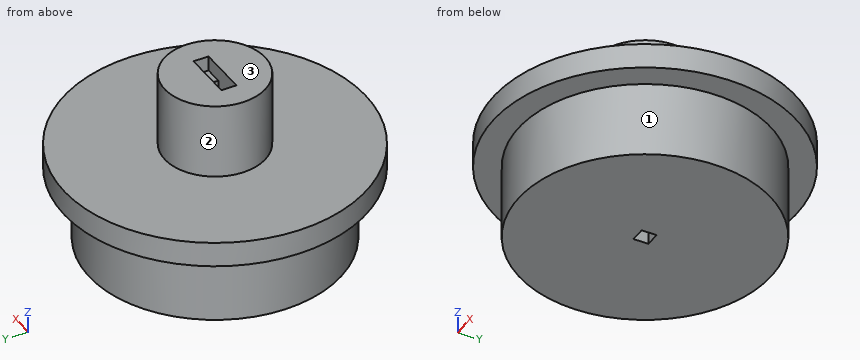
from build123d import *

# Parameters (mm, degrees)
F2_W     = 10
F2_H     = 3
F3_DEPTH = 3
F4_W     = 3
F4_H     = 3
F5_DEPTH = 40


with BuildPart() as f1:
    # F0 (on Front) → F1 (revolve)
    with BuildSketch(Plane.XZ):
        Polygon((0, 13.734525), (-1.5, 13.734525), (-10, 13.734525), (-10, -1.265475), (-25, -1.265475), (-30, -1.265475), (-30, -6.265475), (-25, -6.265475), (-25, -21.265475), (0, -21.265475), (0, 9.622872), align=None)
    revolve(axis=Axis((0, 0, 2.372262), (0, 0, -1)))

    # F2 (on face) → F3 (cut)
    with BuildSketch(Plane.XY.offset(13.734525)):
        Rectangle(F2_W, F2_H)
    extrude(amount=-F3_DEPTH, mode=Mode.SUBTRACT)

    # F4 (on face) → F5 (cut)
    with BuildSketch(Plane.XY.offset(10.734525)):
        Rectangle(F4_W, F4_H)
    extrude(amount=-F5_DEPTH, mode=Mode.SUBTRACT)


solid = f1.part
Can you work these out from the model? Positions are in its coordinate system, mm. Face numbers are marked on the shaded views. A direction names the side the tool comes from. Round coordinates to 2 decimals unless told otherwise and drop trailing zeros. Loops run counter-clockwise (first coordinate to the right, second up) from the corner with the lowest first, then second, coordinate; pieces in that order, holes last. Notation, with made-up numbers: (12.25, 61.5) - (40.25, 61.5) arc R16 ccw to (40.25, 77.5) - close; hole circle Ø6 at (40, 51). An arc over 180 degrees is marked (long way). Answer in a Markdown table with one row per item. Add a question column.
Q1. I need wall thicknesses on L1, parallel to Z at x = 4.5, y = -18.5; L2, parallel to Z at x = -12, y = -24.5; L3, parallel to Y at x = -8.5, z = -16. Which ranges of each line are inside material? Lowest first, please.
Q2. I want a section at B-B on y = 0. List the corners of the cut face in (x, z) for me.
Q3. I want a section at C-C on z = -3. List the corners of the cut face in (x, y) for me.
Q4. For pin 1 Ø0.9 at (x, y) = (-3, 0.5) entering from +Z; pin 2 Ø11 at (x, z) = (-0.5, -11.5) entering from +Y; pin 3 Ø5 at (x, z) = (21, -4) entering from +Y, each with a flat end and sliding along its axis, tell me the tip position at first contact or that it passes through.
Q5. I want a section at A-A on x = 0. List the corners of the cut face in (y, z) for me, and give its area (4 significant figures).
Q6. I want a section at D-D on x = -24. List the corners of the cut face in (y, z) for me.
Q7. Which directions (+Z, -Z, +X, -X, +Y, -Y) give clear straight access to the entire face, cutting with the end or side of a thin tool? Please do the marked faces 1, 2 and 3.
A:
| question | item | result |
|---|---|---|
| 1 | L1 | -21.27 to -1.27 |
| 1 | L2 | -6.27 to -1.27 |
| 1 | L3 | -23.51 to 23.51 |
| 2 | outline | (-30, -6.27) - (-25, -6.27) - (-25, -21.27) - (-1.5, -21.27) - (-1.5, 10.73) - (-5, 10.73) - (-5, 13.73) - (-10, 13.73) - (-10, -1.27) - (-30, -1.27) - close; (1.5, -21.27) - (25, -21.27) - (25, -6.27) - (30, -6.27) - (30, -1.27) - (10, -1.27) - (10, 13.73) - (5, 13.73) - (5, 10.73) - (1.5, 10.73) - close |
| 3 | outline | circle Ø60 at (0, 0); hole (-1.5, -1.5) - (1.5, -1.5) - (1.5, 1.5) - (-1.5, 1.5) - close |
| 4 | pin 1 | z = 10.73 |
| 4 | pin 2 | y = 30 |
| 4 | pin 3 | y = 23.62 |
| 5 | outline | (-30, -6.27) - (-25, -6.27) - (-25, -21.27) - (-1.5, -21.27) - (-1.5, 13.73) - (-10, 13.73) - (-10, -1.27) - (-30, -1.27) - close; (1.5, -21.27) - (25, -21.27) - (25, -6.27) - (30, -6.27) - (30, -1.27) - (10, -1.27) - (10, 13.73) - (1.5, 13.73) - close |
| 5 | area | 1,245 mm^2 |
| 6 | outline | (-18, -6.27) - (-7, -6.27) - (-7, -21.27) - (7, -21.27) - (7, -6.27) - (18, -6.27) - (18, -1.27) - (-18, -1.27) - close |
| 7 | face 1 | -Z |
| 7 | face 2 | +Z |
| 7 | face 3 | +Z, +X, -X, +Y, -Y |
